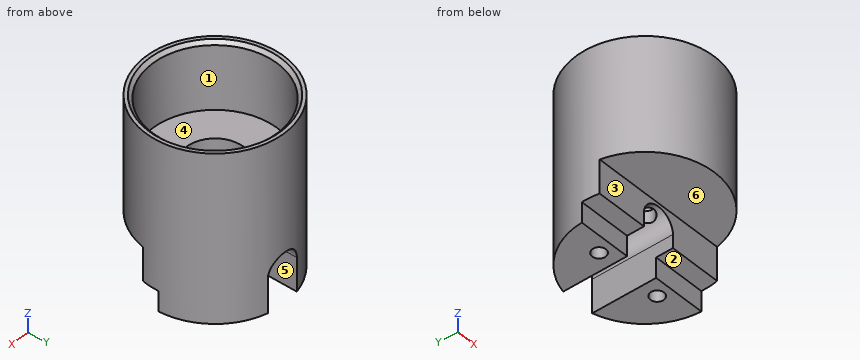
```python
from build123d import *

# Parameters (mm, degrees)
F3_DEPTH  = 18
F4_W      = 8.3
F4_H      = 8
F5_DEPTH  = 10.3
F6_W      = 7.6039596199
F6_H      = 3
F6_W_2    = 0.1960403801
F7_DEPTH  = 2.5
F8_SIZE   = 0.5
F9_R      = 1
F10_DEPTH = 10


# Not quite as in the source:
# - a feature names something its author has since deleted; it is built from what else it names


with BuildPart() as f1:
    # F0 (on Front) → F1 (revolve)
    with BuildSketch(Plane.XZ):
        Polygon((-10.3, 0), (-1.3, 0), (-1.3, 9), (-4.3, 9), (-4.3, 15), (-9.3, 15), (-9.3, 25), (-10.3, 25), align=None)
    revolve(axis=Axis((0, 0, 8.3402672317), (0, 0, 1)))

    # F2 (on Front) → F3 (cut, symmetric)
    with BuildSketch(Plane.XZ):
        with BuildLine():
            Line((-2.5, 5), (-2.5, 0))
            Line((-2.5, 0), (0, 0))
            Line((0, 0), (2.5, 0))
            Line((2.5, 0), (2.5, 5))
            ThreePointArc((2.5, 5), (0, 2.5), (-2.5, 5))
        make_face()
        with BuildLine():
            ThreePointArc((2.5, 5), (0, 7.5), (-2.5, 5))
            ThreePointArc((-2.5, 5), (0, 2.5), (2.5, 5))
        make_face()
    extrude(amount=F3_DEPTH, both=True, mode=Mode.SUBTRACT)

    # F4 (on Right) → F5 (cut, symmetric)
    with BuildSketch(Plane.YZ):
        with Locations((-6.15, 4)):
            Rectangle(F4_W, F4_H)
    extrude(amount=F5_DEPTH, both=True, mode=Mode.SUBTRACT)

    # F6 (on face) → F7 (cut)
    with BuildSketch(Plane.XZ.offset(2)):
        with Locations((6.3019798099, 1.5)):
            Rectangle(F6_W, F6_H)
        with Locations((-6.3019798099, 1.5)):
            Rectangle(F6_W, F6_H)
        with Locations((10.2019798099, 1.5)):
            Rectangle(F6_W_2, F6_H)
        with Locations((-10.2019798099, 1.5)):
            Rectangle(F6_W_2, F6_H)
    extrude(amount=-F7_DEPTH, mode=Mode.SUBTRACT)

    # F8
    f8_edges = [f1.edges().sort_by_distance(p)[0] for p in [
        (9.3, 0, 25),
    ]]
    chamfer(f8_edges, length=F8_SIZE)

    # F9 (on face) → F10 (cut)
    with BuildSketch(Plane(origin=(0, 0, 0), x_dir=(1, 0, 0), z_dir=(0, 0, -1))):
        with Locations((-5, -2.5)):
            Circle(F9_R)
        with Locations((5, -2.5)):
            Circle(F9_R)
    extrude(amount=-F10_DEPTH, mode=Mode.SUBTRACT)


solid = f1.part
```
Model file for the job. Use its own axes, mm. Face numbers are marked on the shaded views. A direction names the side the tool comes from. Round coordinates to 2 decimals unless told otherwise and drop trailing zeros. Loops run counter-clockwise (first coordinate to the right, second up) from the corner with the lowest first, then second, coordinate; pieces in that order, holes last. Notation, with made-up numbers: M -2.5,-33 L 24.5,-33 A29 cw 24.5,3 Z; hole C 32,32.25 d7. An arc over 180 degrees is marked long. Put each result on its own line as item: value. Start each with the question number.
Item 1: Mould opens along Y. For the marked faces 1, 2 and 3 say: released by +Y, released by -Y, zero draft, split by the parting line, or undercut.
Item 2: Drop flat-ended pins along their axis: P1, Ø6, axis at x = -7, z = 14, coming from the +Y side; P2, Ø6, axis at x = -0.5, y = -4, coming from the +Z side; P3, Ø4, axis at x = 0, y = 0, coming from the -Z side; P4, Ø1, axis at x = 5, y = 5, coming from the -Z side. Give the stop position or say it passes through.
Item 3: Cut at B-B (x = 0). List the corners of the cut face in (y, z).
Item 4: Drill centre lines: line 1 along Y through (x, z) = (0, 11.9); line 2 along X through (y, z) = (-0.25, 13); line 3 along Y through (x, z) = (0, 19.5). Where is each one in solid material? Low to high.
Item 5: Cut at A-A (z = 3.75). List the corners of the cut face in (x, y), then the cut area to 3 significant figures.
Item 6: Cut at C-C (y = 0). List the corners of the cut face in (x, z).
Item 7: 3-axis set-ups, long thin cutter, end or side, ignore diameter. For the marked faces 4, 5 and 6: which of +Z, -Z, +X, -X, +Y, -Y reach the whole face in a straight line?
Item 8: Cut at D-D (z = 13). List the corners of the cut face in (x, y).
Answer block:
1. face 1: undercut
1. face 2: zero draft
1. face 3: released by -Y
2. P1: y = 9.49
2. P2: z = 15
2. P3: z = 6.5
2. P4: z = 0
3. outline: M -10.3,8 L -2,8 L -2,7.5 L -1.3,7.5 L -1.3,9 L -4.3,9 L -4.3,15 L -9.3,15 L -9.3,24.5 L -9.8,25 L -10.3,25 Z; M 1.3,7.5 L 10.3,7.5 L 10.3,25 L 9.8,25 L 9.3,24.5 L 9.3,15 L 4.3,15 L 4.3,9 L 1.3,9 Z
4. line 1: -10.3 to -4.3, 4.3 to 10.3
4. line 2: -10.3 to -4.29, 4.29 to 10.3
4. line 3: -10.3 to -9.3, 9.3 to 10.3
5. outline: M -10.1,-2 L -2.5,-2 L -2.5,9.99 A10.3 ccw Z; M 2.5,-2 L 10.1,-2 A10.3 ccw 2.5,9.99 Z; hole C -5,2.5 d2; hole C 5,2.5 d2
5. area: 140 mm2
6. outline: M -10.3,3 L -2.5,3 L -2.5,5 A2.5 cw -1.3,7.14 L -1.3,9 L -4.3,9 L -4.3,15 L -9.3,15 L -9.3,24.5 L -9.8,25 L -10.3,25 Z; M 1.3,7.14 A2.5 cw 2.5,5 L 2.5,3 L 10.3,3 L 10.3,25 L 9.8,25 L 9.3,24.5 L 9.3,15 L 4.3,15 L 4.3,9 L 1.3,9 Z
7. face 4: +Z
7. face 5: -Z, +Y, -Y
7. face 6: -Z, +X, -X, -Y
8. outline: C 0,0 d20.6; hole C 0,0 d8.6
